Design review of the part built by this model. Coordinates are the model's own, in mm. A direction names the side the tool comes from. Give positions to 0.01 mm unless a question says otherwise; leave off trailing zeros. Order: outer loops, then holes, each group sorted by start corner. A loop starts at its lowest first (then second) coordinate and runs counter-clockwise, first axis right, second up. Notation, with made-up numbers: (28, 61.25) -> (61, 61.25) arc R17 cw to (61, 75.25) -> close; hole circle Ø9 at (-18.5, 0). An arc over 180 degrees is marked (long way). One line per item, written item: value. Start each with the question number.
1) For pin 1 (5 mm diameter, centred on y = 5.5, z = -3, fed in from +X); pin 2 (2 mm diameter, centred on x = 20, y = 0.5, fed in from +Z); pin 3 (1.2 mm diameter, centred on x = -18, y = 0, fed in from -Z), all flat-tipped, find the tip position at first contact; note any pin that passes through.
2) Consider section B-B (y = 1). State the section outline as (x, z) points, plus the area to 3 significant figures.
3) Consider section D-D (z = -22). State the section outline as (x, y) points, plus the area to 3 significant figures.
4) The part is to be moulded in two halves that separate along X. For faces 5 (the face through (15.6, 5.89, -31.14)), 6 (the face through (-25, 0, 0)), 7 (the face through (-14.5, 6, 0)), say which applies: released by +X, released by -X, zero draft, split by the parting line, or undercut.
5) Consider section A-A (z = 0). State the section outline as (x, y) points, plus the area to 3 significant figures.
6) Consider section C-C (y = 12.75). State the section outline as (x, z) points.
7) Wall thickness on line 1 along X through (y, z) = (0.6, 0); line 2 along X through (y, z) = (10.75, -5); line 3 along Z through (x, y) = (-13, 9): over which ranges is each line inside the solid? List them lowest first. Write a range as from..to.
8) Tool access review of faces 1 (the face through (19, 2, 0)), 2 (the face through (-19, 2, 0)), 3 (the face through (14.5, 6, 0)), 4 (the face through (-19, 0, -3.5)): name each direction out of +Z, -Z, +X, -X, +Y, -Y from which nothing blocks a thin tool from reaching the whole face with its end or side.
from build123d import *

# Parameters (mm, degrees)
SKETCH2_W           = 33
SKETCH2_H           = 64
SKETCH2_W_2         = 29
SKETCH2_H_2         = 60
BOSS_EXTRUDE1_DEPTH = 14
SKETCH3_W           = 33
SKETCH3_H           = 64
BOSS_EXTRUDE2_DEPTH = 2
SKETCH4_R           = 2.1
BOSS_EXTRUDE3_DEPTH = 4
FILLET1_R           = 3
FILLET2_R           = 2


with BuildPart() as part:
    # Sketch2 → Boss-Extrude1 (new body)
    with BuildSketch(Plane(origin=(0, 0, 0), x_dir=(1, 0, 0), z_dir=(0, 1, 0))):
        Rectangle(SKETCH2_W, SKETCH2_H)
        Rectangle(SKETCH2_W_2, SKETCH2_H_2, mode=Mode.SUBTRACT)
    extrude(amount=BOSS_EXTRUDE1_DEPTH)

    # Sketch3 → Boss-Extrude2 (add)
    with BuildSketch(Plane.XZ):
        Rectangle(SKETCH3_W, SKETCH3_H)
    extrude(amount=BOSS_EXTRUDE2_DEPTH)

    # Sketch4 → Boss-Extrude3 (add)
    # profile 1 of 2: a face of its own
    with BuildSketch(Plane.XZ.offset(2)):
        with BuildLine():
            Line((-21.5, 3.5), (-16.5, 3.5))
            Line((-16.5, 3.5), (-16.5, -3.5))
            Line((-16.5, -3.5), (-21.5, -3.5))
            ThreePointArc((-21.5, -3.5), (-25, 0), (-21.5, 3.5))
        make_face()
        with Locations(Location((-21.5, 0, 0), (0, 0, 270))):
            Circle(SKETCH4_R, mode=Mode.SUBTRACT)
    # profile 2 of 2: a face of its own
    with BuildSketch(Plane.XZ.offset(2)):
        with BuildLine():
            Line((16.5, 3.5), (16.5, -3.5))
            Line((16.5, -3.5), (21.5, -3.5))
            ThreePointArc((21.5, -3.5), (25, 0), (21.5, 3.5))
            Line((21.5, 3.5), (16.5, 3.5))
        make_face()
        with Locations(Location((21.5, 0, 0), (0, 0, 90))):
            Circle(SKETCH4_R, mode=Mode.SUBTRACT)
    extrude(amount=-BOSS_EXTRUDE3_DEPTH)

    # Fillet1
    fillet1_edges = [part.edges().sort_by_distance(p)[0] for p in [
        (16.5, 6, 32),
        (-16.5, 6, 32),
        (-16.5, 6, -32),
        (16.5, 6, -32),
    ]]
    fillet(fillet1_edges, radius=FILLET1_R)

    # Fillet2
    # the kernel refuses this fillet: 2 mm, written as the material it takes off along each edge
    with BuildSketch(Plane(origin=(14.5, 14, -30), x_dir=(1, 0, 0), z_dir=(0, 0, 1)), Plane(origin=(-14.5, 14, 30), x_dir=(-1, 0, 0), z_dir=(0, 0, -1))) as fillet2_piece_1:
        with BuildLine():
            CenterArc((FILLET2_R, -FILLET2_R), FILLET2_R, 90, 90)
            Line((0, -FILLET2_R), (-FILLET2_R * 0.02, -FILLET2_R))
            Line((-FILLET2_R * 0.02, -FILLET2_R), (-FILLET2_R * 0.02, FILLET2_R * 0.02))
            Line((-FILLET2_R * 0.02, FILLET2_R * 0.02), (FILLET2_R, FILLET2_R * 0.02))
            Line((FILLET2_R, FILLET2_R * 0.02), (FILLET2_R, 0))
        make_face()
    extrude(amount=60, mode=Mode.SUBTRACT)
    with BuildSketch(Plane(origin=(-14.5, 14, -30), x_dir=(0, 0, -1), z_dir=(1, 0, 0)), Plane(origin=(14.5, 14, 30), x_dir=(0, 0, 1), z_dir=(-1, 0, 0))) as fillet2_piece_2:
        with BuildLine():
            CenterArc((FILLET2_R, -FILLET2_R), FILLET2_R, 90, 90)
            Line((0, -FILLET2_R), (-FILLET2_R * 0.02, -FILLET2_R))
            Line((-FILLET2_R * 0.02, -FILLET2_R), (-FILLET2_R * 0.02, FILLET2_R * 0.02))
            Line((-FILLET2_R * 0.02, FILLET2_R * 0.02), (FILLET2_R, FILLET2_R * 0.02))
            Line((FILLET2_R, FILLET2_R * 0.02), (FILLET2_R, 0))
        make_face()
    extrude(amount=29, mode=Mode.SUBTRACT)
    with BuildSketch(Plane(origin=(14.5, 14, -35), x_dir=(1, 0, 0), z_dir=(0, 0, 1))) as fillet2_piece_3a_section:
        with BuildLine():
            CenterArc((FILLET2_R, -FILLET2_R), FILLET2_R, 90, 90)
            Line((0, -FILLET2_R), (-FILLET2_R * 0.02, -FILLET2_R))
            Line((-FILLET2_R * 0.02, -FILLET2_R), (-FILLET2_R * 0.02, FILLET2_R * 0.02))
            Line((-FILLET2_R * 0.02, FILLET2_R * 0.02), (FILLET2_R, FILLET2_R * 0.02))
            Line((FILLET2_R, FILLET2_R * 0.02), (FILLET2_R, 0))
        make_face()
    fillet2_piece_3a = extrude(amount=65, mode=Mode.PRIVATE)
    fillet2_piece_3a = split(fillet2_piece_3a, bisect_by=Plane(origin=(14.952790229, 13.547209771, -30), z_dir=(0, 0, -1)), keep=Keep.TOP, mode=Mode.PRIVATE)
    with BuildSketch(Plane(origin=(-14.5, 14, -30), x_dir=(0, 0, -1), z_dir=(1, 0, 0))) as fillet2_piece_3b_section:
        with BuildLine():
            CenterArc((FILLET2_R, -FILLET2_R), FILLET2_R, 90, 90)
            Line((0, -FILLET2_R), (-FILLET2_R * 0.02, -FILLET2_R))
            Line((-FILLET2_R * 0.02, -FILLET2_R), (-FILLET2_R * 0.02, FILLET2_R * 0.02))
            Line((-FILLET2_R * 0.02, FILLET2_R * 0.02), (FILLET2_R, FILLET2_R * 0.02))
            Line((FILLET2_R, FILLET2_R * 0.02), (FILLET2_R, 0))
        make_face()
    fillet2_piece_3b = extrude(amount=34, mode=Mode.PRIVATE)
    fillet2_piece_3b = split(fillet2_piece_3b, bisect_by=Plane(origin=(14.5, 13.547209771, -30.452790229), z_dir=(1, 0, 0)), keep=Keep.TOP, mode=Mode.PRIVATE)
    fillet2_piece_3 = fillet2_piece_3a & fillet2_piece_3b
    add(fillet2_piece_3, mode=Mode.SUBTRACT)
    with BuildSketch(Plane(origin=(19.5, 14, 30), x_dir=(0, 0, 1), z_dir=(-1, 0, 0))) as fillet2_piece_4a_section:
        with BuildLine():
            CenterArc((FILLET2_R, -FILLET2_R), FILLET2_R, 90, 90)
            Line((0, -FILLET2_R), (-FILLET2_R * 0.02, -FILLET2_R))
            Line((-FILLET2_R * 0.02, -FILLET2_R), (-FILLET2_R * 0.02, FILLET2_R * 0.02))
            Line((-FILLET2_R * 0.02, FILLET2_R * 0.02), (FILLET2_R, FILLET2_R * 0.02))
            Line((FILLET2_R, FILLET2_R * 0.02), (FILLET2_R, 0))
        make_face()
    fillet2_piece_4a = extrude(amount=34, mode=Mode.PRIVATE)
    fillet2_piece_4a = split(fillet2_piece_4a, bisect_by=Plane(origin=(14.5, 13.547209771, 30.452790229), z_dir=(1, 0, 0)), keep=Keep.TOP, mode=Mode.PRIVATE)
    with BuildSketch(Plane(origin=(14.5, 14, -30), x_dir=(1, 0, 0), z_dir=(0, 0, 1))) as fillet2_piece_4b_section:
        with BuildLine():
            CenterArc((FILLET2_R, -FILLET2_R), FILLET2_R, 90, 90)
            Line((0, -FILLET2_R), (-FILLET2_R * 0.02, -FILLET2_R))
            Line((-FILLET2_R * 0.02, -FILLET2_R), (-FILLET2_R * 0.02, FILLET2_R * 0.02))
            Line((-FILLET2_R * 0.02, FILLET2_R * 0.02), (FILLET2_R, FILLET2_R * 0.02))
            Line((FILLET2_R, FILLET2_R * 0.02), (FILLET2_R, 0))
        make_face()
    fillet2_piece_4b = extrude(amount=65, mode=Mode.PRIVATE)
    fillet2_piece_4b = split(fillet2_piece_4b, bisect_by=Plane(origin=(14.952790229, 13.547209771, 30), z_dir=(0, 0, 1)), keep=Keep.TOP, mode=Mode.PRIVATE)
    fillet2_piece_4 = fillet2_piece_4a & fillet2_piece_4b
    add(fillet2_piece_4, mode=Mode.SUBTRACT)
    with BuildSketch(Plane(origin=(-14.5, 14, 30), x_dir=(-1, 0, 0), z_dir=(0, 0, -1))) as fillet2_piece_5a_section:
        with BuildLine():
            CenterArc((FILLET2_R, -FILLET2_R), FILLET2_R, 90, 90)
            Line((0, -FILLET2_R), (-FILLET2_R * 0.02, -FILLET2_R))
            Line((-FILLET2_R * 0.02, -FILLET2_R), (-FILLET2_R * 0.02, FILLET2_R * 0.02))
            Line((-FILLET2_R * 0.02, FILLET2_R * 0.02), (FILLET2_R, FILLET2_R * 0.02))
            Line((FILLET2_R, FILLET2_R * 0.02), (FILLET2_R, 0))
        make_face()
    fillet2_piece_5a = extrude(amount=65, mode=Mode.PRIVATE)
    fillet2_piece_5a = split(fillet2_piece_5a, bisect_by=Plane(origin=(-14.952790229, 13.547209771, -30), z_dir=(0, 0, -1)), keep=Keep.TOP, mode=Mode.PRIVATE)
    with BuildSketch(Plane(origin=(-19.5, 14, -30), x_dir=(0, 0, -1), z_dir=(1, 0, 0))) as fillet2_piece_5b_section:
        with BuildLine():
            CenterArc((FILLET2_R, -FILLET2_R), FILLET2_R, 90, 90)
            Line((0, -FILLET2_R), (-FILLET2_R * 0.02, -FILLET2_R))
            Line((-FILLET2_R * 0.02, -FILLET2_R), (-FILLET2_R * 0.02, FILLET2_R * 0.02))
            Line((-FILLET2_R * 0.02, FILLET2_R * 0.02), (FILLET2_R, FILLET2_R * 0.02))
            Line((FILLET2_R, FILLET2_R * 0.02), (FILLET2_R, 0))
        make_face()
    fillet2_piece_5b = extrude(amount=34, mode=Mode.PRIVATE)
    fillet2_piece_5b = split(fillet2_piece_5b, bisect_by=Plane(origin=(-14.5, 13.547209771, -30.452790229), z_dir=(-1, 0, 0)), keep=Keep.TOP, mode=Mode.PRIVATE)
    fillet2_piece_5 = fillet2_piece_5a & fillet2_piece_5b
    add(fillet2_piece_5, mode=Mode.SUBTRACT)
    with BuildSketch(Plane(origin=(-14.5, 14, 35), x_dir=(-1, 0, 0), z_dir=(0, 0, -1))) as fillet2_piece_6a_section:
        with BuildLine():
            CenterArc((FILLET2_R, -FILLET2_R), FILLET2_R, 90, 90)
            Line((0, -FILLET2_R), (-FILLET2_R * 0.02, -FILLET2_R))
            Line((-FILLET2_R * 0.02, -FILLET2_R), (-FILLET2_R * 0.02, FILLET2_R * 0.02))
            Line((-FILLET2_R * 0.02, FILLET2_R * 0.02), (FILLET2_R, FILLET2_R * 0.02))
            Line((FILLET2_R, FILLET2_R * 0.02), (FILLET2_R, 0))
        make_face()
    fillet2_piece_6a = extrude(amount=65, mode=Mode.PRIVATE)
    fillet2_piece_6a = split(fillet2_piece_6a, bisect_by=Plane(origin=(-14.952790229, 13.547209771, 30), z_dir=(0, 0, 1)), keep=Keep.TOP, mode=Mode.PRIVATE)
    with BuildSketch(Plane(origin=(14.5, 14, 30), x_dir=(0, 0, 1), z_dir=(-1, 0, 0))) as fillet2_piece_6b_section:
        with BuildLine():
            CenterArc((FILLET2_R, -FILLET2_R), FILLET2_R, 90, 90)
            Line((0, -FILLET2_R), (-FILLET2_R * 0.02, -FILLET2_R))
            Line((-FILLET2_R * 0.02, -FILLET2_R), (-FILLET2_R * 0.02, FILLET2_R * 0.02))
            Line((-FILLET2_R * 0.02, FILLET2_R * 0.02), (FILLET2_R, FILLET2_R * 0.02))
            Line((FILLET2_R, FILLET2_R * 0.02), (FILLET2_R, 0))
        make_face()
    fillet2_piece_6b = extrude(amount=34, mode=Mode.PRIVATE)
    fillet2_piece_6b = split(fillet2_piece_6b, bisect_by=Plane(origin=(-14.5, 13.547209771, 30.452790229), z_dir=(-1, 0, 0)), keep=Keep.TOP, mode=Mode.PRIVATE)
    fillet2_piece_6 = fillet2_piece_6a & fillet2_piece_6b
    add(fillet2_piece_6, mode=Mode.SUBTRACT)


solid = part.part
Checked values:
1. pin 1: stops at x = 16.5
1. pin 2: stops at z = 3.5
1. pin 3: stops at z = -3.5
2. outline: (-21.5, -3.5) -> (-16.5, -3.5) -> (-16.5, -29) arc R3 ccw to (-13.5, -32) -> (13.5, -32) arc R3 ccw to (16.5, -29) -> (16.5, -3.5) -> (21.5, -3.5) arc R3.5 ccw to (21.5, 3.5) -> (16.5, 3.5) -> (16.5, 29) arc R3 ccw to (13.5, 32) -> (-13.5, 32) arc R3 ccw to (-16.5, 29) -> (-16.5, 3.5) -> (-21.5, 3.5) arc R3.5 ccw to start; hole circle Ø4.2 at (-21.5, 0); hole (-14.5, -30) -> (14.5, -30) -> (14.5, 30) -> (-14.5, 30) -> close; hole circle Ø4.2 at (21.5, 0)
2. area: 445 mm^2
3. outline: (-16.5, -2) -> (16.5, -2) -> (16.5, 14) arc R2 ccw to (14.5, 12) -> (14.5, 0) -> (-14.5, 0) -> (-14.5, 12) arc R2 ccw to (-16.5, 14) -> close
3. area: 120 mm^2
4. face 5: released by +X
4. face 6: released by -X
4. face 7: undercut
5. outline: (-25, -2) -> (-23.6, -2) -> (-23.6, 2) -> (-25, 2) -> close; (-19.4, -2) -> (19.4, -2) -> (19.4, 2) -> (16.5, 2) -> (16.5, 14) arc R2 ccw to (14.5, 12) -> (14.5, 0) -> (-14.5, 0) -> (-14.5, 12) arc R2 ccw to (-16.5, 14) -> (-16.5, 2) -> (-19.4, 2) -> close; (23.6, -2) -> (25, -2) -> (25, 2) -> (23.6, 2) -> close
5. area: 155 mm^2
6. outline: (-16.5, -29) arc R3 ccw to (-13.5, -32) -> (13.5, -32) arc R3 ccw to (16.5, -29) -> (16.5, 29) arc R3 ccw to (13.5, 32) -> (-13.5, 32) arc R3 ccw to (-16.5, 29) -> close; hole (-14.65, -30.15) -> (14.65, -30.15) -> (14.65, 30.15) -> (-14.65, 30.15) -> close
7. line 1: x = -25..-23.6, -19.4..-14.5, 14.5..19.4, 23.6..25
7. line 2: x = -16.5..-14.5, 14.5..16.5
7. line 3: z = -32..-30, 30..32
8. face 1: +Z, -Z, +X, +Y
8. face 2: +Z, -Z, -X, +Y
8. face 3: +Y
8. face 4: -Z, -X, +Y, -Y
